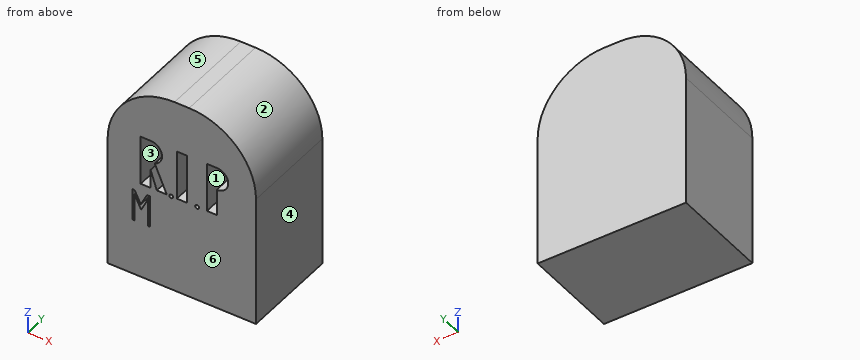
from build123d import *

# Parameters (mm, degrees)
F0_W      = 38.1
F0_H      = 25.4
F1_DEPTH  = 50.8
F2_R      = 17.169887
F4_DEPTH  = 12.7
F7_DEPTH  = 12.7
F9_DEPTH  = 12.7
F10_R     = 0.493061
F11_DEPTH = 12.7
F14_DEPTH = 12.7


with BuildPart() as f1:
    # F0 (on Top) → F1 (new body)
    with BuildSketch(Plane.XY):
        Rectangle(F0_W, F0_H)
    extrude(amount=F1_DEPTH)

    # F2
    f2_edges = [f1.edges().sort_by_distance(p)[0] for p in [
        (19.05, 0, 50.8),
        (-19.05, 0, 50.8),
    ]]
    fillet(f2_edges, radius=F2_R)

    # F3 (on face) → F4 (cut)
    with BuildSketch(Plane.XZ.offset(12.7)):
        Polygon((1.27, 25.041066), (1.27, 37.741066), (-1.27, 37.741066), (-1.27, 25.041066), (0, 25.041066), align=None)
    extrude(amount=-F4_DEPTH, mode=Mode.SUBTRACT)

    # F6 (on face) → F7 (cut)
    with BuildSketch(Plane.XZ.offset(12.7)):
        Polygon((6.439812, 37.741066), (6.439812, 25.041066), (8.979812, 25.041066), (8.979812, 31.852105), (8.979812, 37.741066), align=None)
        with BuildLine():
            ThreePointArc((8.979812, 31.852105), (11.924293, 34.796585), (8.979812, 37.741066))
            Line((8.979812, 37.741066), (8.979812, 31.852105))
        make_face()
    extrude(amount=-F7_DEPTH, mode=Mode.SUBTRACT)

    # F8 (on face) → F9 (cut)
    with BuildSketch(Plane.XZ.offset(12.7)):
        Polygon((-10.559579, 37.741066), (-10.559579, 25.041066), (-8.019579, 25.041066), (-8.019579, 29.893864), (-8.019579, 31.852105), (-8.019579, 37.741066), align=None)
        with BuildLine():
            Line((-8.019579, 31.852105), (-8.019579, 29.893864))
            Line((-8.019579, 29.893864), (-6.416946, 25.041066))
            Line((-6.416946, 25.041066), (-3.876946, 25.041066))
            Line((-3.876946, 25.041066), (-6.945879, 32.054846))
            ThreePointArc((-6.945879, 32.054846), (-7.473242, 31.903234), (-8.019579, 31.852105))
        make_face()
        with BuildLine():
            ThreePointArc((-6.945879, 32.054846), (-5.126227, 35.342922), (-8.019579, 37.741066))
            Line((-8.019579, 37.741066), (-8.019579, 31.852105))
            ThreePointArc((-8.019579, 31.852105), (-7.473242, 31.903234), (-6.945879, 32.054846))
        make_face()
    extrude(amount=-F9_DEPTH, mode=Mode.SUBTRACT)

    # F10 (on face) → F11 (cut)
    with BuildSketch(Plane.XZ.offset(12.7)):
        with Locations((-2.736643, 25.041066)):
            Circle(F10_R)
        with Locations((3.919682, 25.041066)):
            Circle(F10_R)
    extrude(amount=-F11_DEPTH, mode=Mode.SUBTRACT)

    # F13 (on face) → F14 (cut)
    with BuildSketch(Plane.XZ.offset(12.7)):
        Polygon((-12.685429, 22.705782), (-12.685429, 14.469298), (-12.164247, 14.469298), (-12.164247, 21.557376), (-10.444346, 18.105285), (-8.724445, 21.557376), (-8.724445, 14.469298), (-8.203262, 14.469298), (-8.203262, 22.705782), (-8.946966, 22.705782), (-10.543204, 19.501902), (-12.139441, 22.705782), align=None)
    extrude(amount=-F14_DEPTH, mode=Mode.SUBTRACT)


solid = f1.part
Design review of the part built by this model. Coordinates are the model's own, in mm. Face numbers are marked on the shaded views. A direction names the side the tool comes from. Coordinates: 2 decimals unless noted, no trailing zeros. Write each loop counter-clockwise with the first axis right and the second up, starting at its lowest first coordinate (ties: lowest second). Pieces come first, ordered by that corner, then holes. Notation, with made-up numbers: (86.25, -3) - (140.25, -3) arc R34 ccw to (140.25, 36) - close; hole circle Ø5 at (84.5, 83). An arc over 180 degrees is marked (long way). Use one line per item in the form item = value.
Q1. Insertion check: pin 1 Ø1.3 at (x, y) = (-9, -6) entering from +Z; pin 2 Ø1.5 at (x, y) = (-11.5, -4.5) entering from +Z. Each pin has a flat end and moves straight along its axis. Give the tip position at first contact, or say it passes through.
Taken from the geometry:
pin_1 = 49.53
pin_2 = 48.33
Q2. Machinability: for the marked faces 1 and 2, which of the approach directions +Z, -Z, +X, -X, +Y, -Y give a long, thin tool a straight path to every point of the face, cutting with its end or side? Answer none if there is none.
Taken from the geometry:
face_1 = -Y
face_2 = +Z, +X, +Y, -Y
Q3. The part is to be moulded in two halves that separate along X. For the marked faces 3, 4, 5 and 6, say which applies: +X half, -X half, draft (parallel to the pull), parting line (faces both ways), or undercut.
Taken from the geometry:
face_3 = undercut
face_4 = +X half
face_5 = -X half
face_6 = draft
Q4. For probe 1 along X at (y, z) = (-6.75, 28); probe 2 along Z at (x, y) = (-10.5, -10.25); probe 3 along Z at (x, y) = (-2, 5.5), list the stretches that pass through material, from the lowest coordinate up.
Taken from the geometry:
probe_1 = -19.05 to -10.56, -8.02 to -7.39, -5.17 to -1.27, 1.27 to 6.44, 8.98 to 19.05
probe_2 = 0 to 18.22, 19.59 to 25.04, 37.74 to 48.48
probe_3 = 0 to 50.8
Q5. Consider section B-B (z = 36.5). Write out the cut boundary in (x, y).
Taken from the geometry:
outline = (-18.81, -12.7) - (-10.56, -12.7) - (-10.56, 0) - (-5.62, 0) - (-5.62, -12.7) - (-1.27, -12.7) - (-1.27, 0) - (1.27, 0) - (1.27, -12.7) - (6.44, -12.7) - (6.44, 0) - (11.38, 0) - (11.38, -12.7) - (18.81, -12.7) - (18.81, 12.7) - (-18.81, 12.7) - close
Q6. Consider section C-C (x = 7.5). Write out the cut boundary in (y, z).
Taken from the geometry:
outline = (-12.7, 0) - (12.7, 0) - (12.7, 49.85) - (-12.7, 49.85) - (-12.7, 37.74) - (0, 37.74) - (0, 25.04) - (-12.7, 25.04) - close
Q7. Consider section A-A (y = -1.25). Count the separate pieces of the cut face and the enclosed holes in it, plus the area to 3 significant figures.
Taken from the geometry:
separate_pieces = 1
enclosed_holes = 6
area = 1,660 mm^2
Q8. Consider section D-D (y = 9). Write out the cut boundary in (x, z), plus the area to 3 significant figures.
Taken from the geometry:
outline = (-19.05, 0) - (19.05, 0) - (19.05, 33.63) arc R17.17 ccw to (1.88, 50.8) - (-1.88, 50.8) arc R17.17 ccw to (-19.05, 33.63) - close
area = 1,810 mm^2
